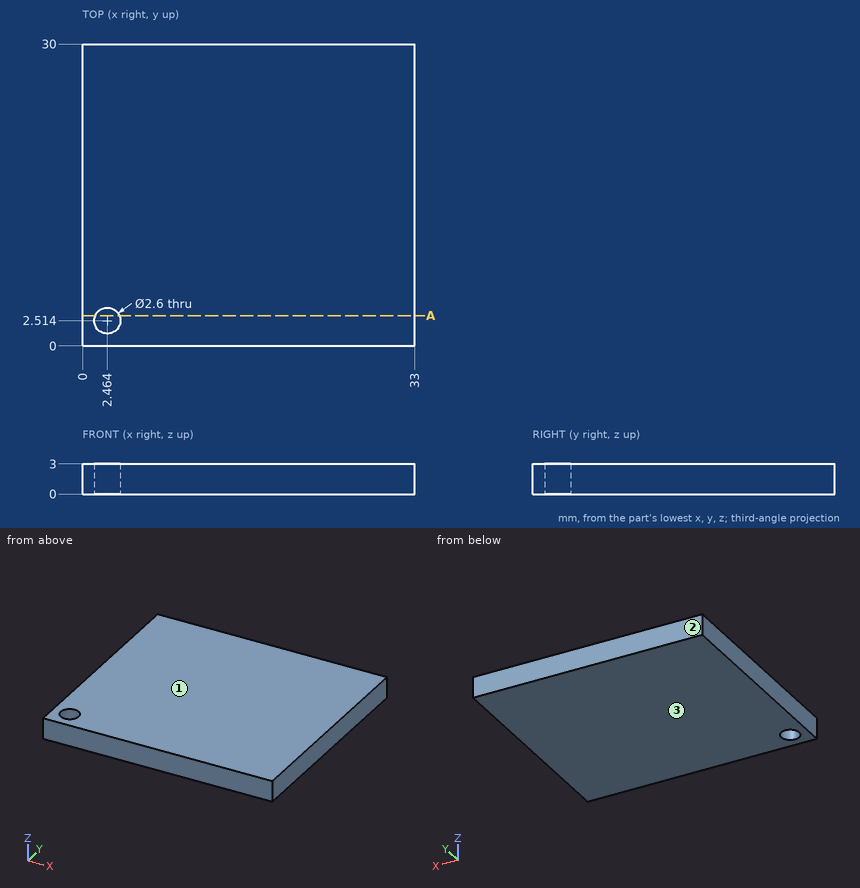
Input: dimensioned drawing with shaded views. Units: mm. Origin: part minimum x, y, z. Coordinates: 2 decimals unless noted, no trailing zeros. Order: outer loops, then holes, each group sorted by start corner. A loop starts at its lowest first (then second) coordinate and runs counter-clockwise, first axis right, second up. Notation, with made-up numbers: (84, 22) - (130, 22) arc R23 cw to (130, 45) - close; hole circle Ø9 at (-32.5, 6.25). An arc over 180 degrees is marked (long way). One line per item, written item: value.
1) Ray query, line 1 (X direction, y = 1.5, z = 1.5). Return the intervals inside material, ascending. Write a range as [from, to].
Computed values:
line 1: x = [0, 1.65], [3.28, 33]
2) Mould query, pull axis Z, two halves, no side actions, for the marked faces 1, 2 and 3. Classes: released by +Z, released by -Z, zero draft, split by the parting line, or undercut.
Computed values:
face 1: released by +Z
face 2: zero draft
face 3: released by -Z
3) Cut plane A-A on y = 3. Output: boundary loops of the cut face in (x, z).
Computed values:
outline: (0, 0) - (1.26, 0) - (1.26, 3) - (0, 3) - close; (3.67, 0) - (33, 0) - (33, 3) - (3.67, 3) - close
4) Contact query for flat-ended pins moving along their axis: pin 1 (1.5 mm diameter, centred on y = 22, z = 0.5, fed in from -X); pin 2 (2.5 mm diameter, centred on x = 2.46, y = 2.51, fed in from +Z). Output: stop coordinate, or through.
Computed values:
pin 1: stops at x = 0
pin 2: passes through
